```python
from build123d import *

# Parameters (mm, degrees)
SKETCH2_R           = 2.5
BOSS_EXTRUDE1_DEPTH = 5
SKETCH4_R           = 2.5
SKETCH4_R_2         = 0.5
BOSS_EXTRUDE3_DEPTH = 8


with BuildPart() as part:
    # Sketch2 → Boss-Extrude1 (new body)
    with BuildSketch(Plane.XY):
        with BuildLine():
            Line((-58.980456911, 11.76034449), (0.519543089, 3.966115855))
            ThreePointArc((0.519543089, 3.966115855), (1.767996055, 3.588062144), (2.828427125, 2.828427125))
            Line((2.828427125, 2.828427125), (15.556349186, -9.899494937))
            ThreePointArc((15.556349186, -9.899494937), (16.265540761, -14.594805544), (11.989145433, -16.659106246))
            Line((11.989145433, -16.659106246), (-55.738776628, -3.931184185))
            ThreePointArc((-55.738776628, -3.931184185), (-57.312663934, -3.263676689), (-58.464101615, -2))
            Line((-58.464101615, -2), (-62.964101615, 5.794228634))
            ThreePointArc((-62.964101615, 5.794228634), (-62.826595982, 10.015435327), (-58.980456911, 11.76034449))
        make_face()
        with Locations((-55, 0)):
            Circle(SKETCH2_R, mode=Mode.SUBTRACT)
        with Locations((-59.5, 7.794228634)):
            Circle(SKETCH2_R, mode=Mode.SUBTRACT)
        Circle(SKETCH2_R, mode=Mode.SUBTRACT)
        with Locations((12.727922061, -12.727922061)):
            Circle(SKETCH2_R, mode=Mode.SUBTRACT)
    extrude(amount=BOSS_EXTRUDE1_DEPTH)

    # Sketch4 → Boss-Extrude3 (add)
    # profile 1 of 2: a face of its own
    with BuildSketch(Plane(origin=(0, 0, 0), x_dir=(-1, 0, 0), z_dir=(0, 0, -1))):
        with Locations((59.5, 7.794228634)):
            Circle(SKETCH4_R)
        with Locations((59.5, 7.794228634)):
            Circle(SKETCH4_R_2, mode=Mode.SUBTRACT)
    # profile 2 of 2: a face of its own
    with BuildSketch(Plane(origin=(0, 0, 0), x_dir=(-1, 0, 0), z_dir=(0, 0, -1))):
        with Locations((-12.727922061, -12.727922061)):
            Circle(SKETCH4_R)
        with Locations((-12.727922061, -12.727922061)):
            Circle(SKETCH4_R_2, mode=Mode.SUBTRACT)
    extrude(amount=-BOSS_EXTRUDE3_DEPTH)


solid = part.part
```
Geometry check sheet. Reference: the model listing, model coordinates, mm. A direction names the side the tool comes from. Coordinates: 2 decimals unless noted, no trailing zeros. Order: outer loops, then holes, each group sorted by start corner. A loop starts at its lowest first (then second) coordinate and runs counter-clockwise, first axis right, second up. Notation, with made-up numbers: (72.25, 81) - (104.25, 81) arc R20 ccw to (104.25, 103) - close; hole circle Ø3 at (68.25, 41.25). An arc over 180 degrees is marked (long way). Answer in a Markdown table with one row per item. Add a question column.
1. Section check B-B (z = 7). Enter the section's corners in (x, y).
2. Access from +Z, -Z, +X, -X, +Y, -Y to the whole of each face (thin tool, end or side, straight path). Record for faces 4 (the face through (1.752, 3.596, 2.465)), 5 (the face through (-61.9, 8.5, 6.5)).
3. Section check D-D (z = 3.5). Enter the section's corners in (x, y).
4. Section check C-C (y = -1). Enter the section's corners in (x, z).
5. Section check A-A (x = -55). Enter the section's corners in (y, z).
6. Draft check along X on faces 1 (the face through (-0.54, -2.44, 2.46)), 2 (the face through (-23, -2, 0)), 3 (the face through (9.103, -3.446, 2.465)). Enter one of: +X half, -X half, draft (parallel to the pull), parting line (faces both ways), or undercut.
7. Gauge pin test, flat ends, axial feed: pin 1 Ø8.5 at (x, y) = (-20, 2.5) entering from +Z; pin 2 Ø3 at (x, y) = (-55, 0) entering from +Z; pin 3 Ø2 at (x, z) = (-14, 3.5) entering from +Y; pin 4 Ø2 at (x, z) = (-7.5, 3) entering from +Y. Record the tip position at first contact, or that the pin passes through.
8. Material ranges on L1, parallel to Y at x = -59.5, z = 5.5; L2, parallel to X at y = -12.75, z = 7.75; L3, parallel to Z at x = -47.5, y = -1.25, recorded low to high. Write a range as [from, to].
Data:
| question | item | result |
|---|---|---|
| 1 | outline | circle Ø5 at (-59.5, 7.79); circle Ø5 at (12.73, -12.73); hole circle Ø1 at (-59.5, 7.79); hole circle Ø1 at (12.73, -12.73) |
| 2 | face 4 | +Z, -Z, +X, +Y |
| 2 | face 5 | +Z |
| 3 | outline | (-62.96, 5.79) - (-58.46, -2) arc R4 ccw to (-55.74, -3.93) - (11.99, -16.66) arc R4 ccw to (15.56, -9.9) - (2.83, 2.83) arc R4 ccw to (0.52, 3.97) - (-58.98, 11.76) arc R4 ccw to start; hole circle Ø1 at (-59.5, 7.79); hole circle Ø5 at (-55, 0); hole circle Ø5 at (0, 0); hole circle Ø1 at (12.73, -12.73) |
| 4 | outline | (-59.04, 0) - (-57.29, 0) - (-57.29, 5) - (-59.04, 5) - close; (-52.71, 0) - (-2.29, 0) - (-2.29, 5) - (-52.71, 5) - close; (2.29, 0) - (6.66, 0) - (6.66, 5) - (2.29, 5) - close |
| 5 | outline | (-4.07, 0) - (-2.5, 0) - (-2.5, 5) - (-4.07, 5) - close; (2.5, 0) - (11.24, 0) - (11.24, 5) - (2.5, 5) - close |
| 6 | face 1 | undercut |
| 6 | face 2 | draft |
| 6 | face 3 | +X half |
| 7 | pin 1 | stops at z = 5 |
| 7 | pin 2 | passes through |
| 7 | pin 3 | stops at y = 6 |
| 7 | pin 4 | stops at y = 5.15 |
| 8 | L1 | y = [5.29, 7.29], [8.29, 10.29] |
| 8 | L2 | x = [10.23, 12.23], [13.23, 15.23] |
| 8 | L3 | z = [0, 5] |
